Could you check a few things on this model? Use its own coordinates, in mm. A direction names the side the tool comes from. Coordinates: 2 decimals unless noted, no trailing zeros. Loops run counter-clockwise (first coordinate to the right, second up) from the corner with the lowest first, then second, coordinate; pieces in that order, holes last. Notation, with made-up numbers: (81, -3.75) - (126, -3.75) arc R29 cw to (126, 22.25) - close; hole circle Ø11 at (-32.5, 71.5). An arc over 180 degrees is marked (long way). One line per question, with ' | ' between items. Start each with the question number.
1. Which directions (+Z, -Z, +X, -X, +Y, -Y) give clear straight access to the entire face, cutting with the end or side of a thin tool? Please do faces 4 (the cylindrical face through (-3, -8, 0)), 5 (the cylindrical face through (-1.4, -3.99, -0.06)), 6 (the cylindrical face through (0, 9, 2)), 7 (the flat face through (1, -10.55, -1)).
2. I want a section at D-D, the plane y = -7. Write out the boundary of the cut face in (x, z), then the cut area to 3 significant figures.
3. I want a section at C-C, the plane y = 0.25. Write out the boundary of the cut face in (x, z), then the cut area to 3 significant figures.
4. I want a section at A-A, the plane x = 0. Write out the boundary of the cut face in (y, z), then the cut area to 3 significant figures.
5. I'm going to push flat-ended pins straight in: P1, Ø1, axis at x = 1.5, y = 4, coming from the -Z side; P2, Ø1.5, axis at x = -1.5, y = -4.5, coming from the -Z side; P3, Ø2, axis at x = -1, y = -5, coming from the -Z side. Where does each tip first touch, or does it pass through?
6. We'd pull the mould along X, two halves only. Please class faces 1 (the cylindrical face through (0, -2, 1)), 2 (the flat face through (0, -2.95, 2)), 3 (the cylindrical face through (3.233, 3.641, 1.341)): pulls with the +X half, pulls with the -X half, needs draft (parallel to the pull), parting line crosses it, or undercut.
7. Please list where these lines run through material, in increasing order: L1, parallel to Z at x = 0, y = 7.95; L2, parallel to X at y = -1, z = 0; L3, parallel to Z at x = 0, y = -4. Write a range as [from, to].
8. I want a section at B-B, the plane z = 0. Write out the boundary of the cut face in (x, y), then the cut area to 3 significant figures.
from build123d import *

# Parameters (mm, degrees)
CHAMFER1_SIZE = 0.5


with BuildPart() as part:
    # Sketch1 → Revolve1 (revolve)
    with BuildSketch(Plane.XY):
        Polygon((1, -10.55), (3, -10.55), (3, -5.05), (1.4, -5.05), (1.4, -2.95), (3.5, -2.95), (3.5, 10.55), (2, 10.55), (2, 6.55), (1, 5.972649731), align=None)
    revolve(axis=Axis((0, -10.55, 0), (0, 1, 0)))

    # Chamfer1
    chamfer1_edges = [part.edges().sort_by_distance(p)[0] for p in [
        (-3.5, 10.55, 0),
    ]]
    chamfer(chamfer1_edges, length=CHAMFER1_SIZE)


solid = part.part
Results are:
1) face 4: -Y | face 5: none | face 6: +Y | face 7: +Z, -Z, +X, -X, -Y
2) outline: circle Ø6 at (0, 0); hole circle Ø2 at (0, 0) | area: 25.1 mm2
3) outline: circle Ø7 at (0, 0); hole circle Ø2 at (0, 0) | area: 35.3 mm2
4) outline: (-10.55, -3) - (-5.05, -3) - (-5.05, -1.4) - (-2.95, -1.4) - (-2.95, -3.5) - (10.05, -3.5) - (10.55, -3) - (10.55, -2) - (6.55, -2) - (5.97, -1) - (-10.55, -1) - close; (-10.55, 1) - (5.97, 1) - (6.55, 2) - (10.55, 2) - (10.55, 3) - (10.05, 3.5) - (-2.95, 3.5) - (-2.95, 1.4) - (-5.05, 1.4) - (-5.05, 3) - (-10.55, 3) - close | area: 82.4 mm2
5) P1: stops at z = -3.35 | P2: stops at z = -2.83 | P3: stops at z = -3
6) face 1: undercut | face 2: needs draft | face 3: parting line crosses it
7) L1: z = [-3.5, -2], [2, 3.5] | L2: x = [-3.5, -1], [1, 3.5] | L3: z = [-1.4, -1], [1, 1.4]
8) outline: (-3.5, -2.95) - (-1.4, -2.95) - (-1.4, -5.05) - (-3, -5.05) - (-3, -10.55) - (-1, -10.55) - (-1, 5.97) - (-2, 6.55) - (-2, 10.55) - (-3, 10.55) - (-3.5, 10.05) - close; (1, -10.55) - (3, -10.55) - (3, -5.05) - (1.4, -5.05) - (1.4, -2.95) - (3.5, -2.95) - (3.5, 10.05) - (3, 10.55) - (2, 10.55) - (2, 6.55) - (1, 5.97) - close | area: 82.4 mm2
